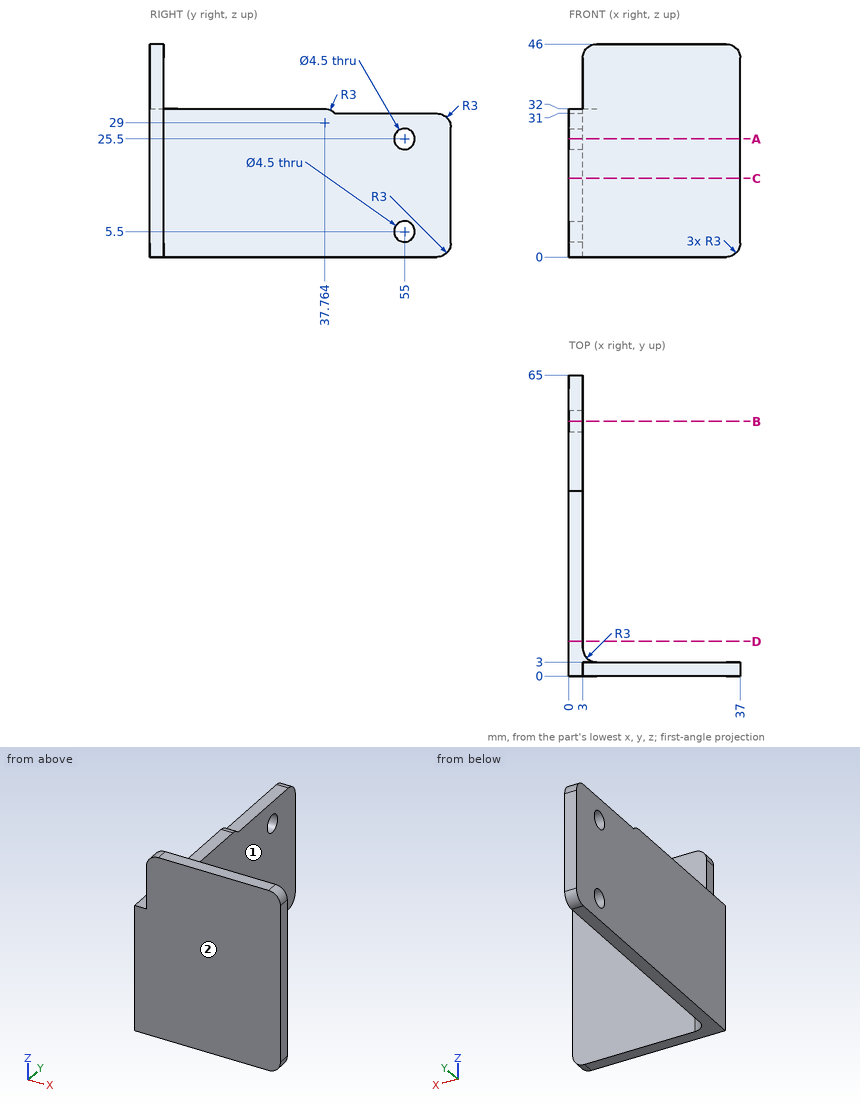
The drawing under review shows one solid part. Ordinate dimensions are in mm from its lowest x, y, z. A direction names the side the tool comes from. Coordinates: 2 decimals unless noted, no trailing zeros. Order: outer loops, then holes, each group sorted by start corner. A loop starts at its lowest first (then second) coordinate and runs counter-clockwise, first axis right, second up. Notation, with made-up numbers: (32.25, -22.75) -> (69.25, -22.75) arc R28 ccw to (69.25, 3.25) -> close; hole circle Ø8 at (-39.75, 23.25). An arc over 180 degrees is marked (long way). Answer as CSV lines item,"result".
Q1. We need section B-B (y = 55). State the section outline as (x, z) points.
Model answer:
outline,"(0, 0) -> (3, 0) -> (3, 3.25) -> (0, 3.25) -> close; (0, 7.75) -> (3, 7.75) -> (3, 23.25) -> (0, 23.25) -> close; (0, 27.75) -> (3, 27.75) -> (3, 31) -> (0, 31) -> close"
Q2. We need section D-D (y = 7.5). State the section outline as (x, z) points, plus the area to 3 significant figures.
Model answer:
outline,"(0, 0) -> (3, 0) -> (3, 32) -> (0, 32) -> close"
area,"96.0 mm2"
Q3. We need section C-C (z = 17). State the section outline as (x, y) points, plus the area to 3 significant figures.
Model answer:
outline,"(0, 0) -> (37, 0) -> (37, 3) -> (6, 3) arc R3 cw to (3, 6) -> (3, 65) -> (0, 65) -> close"
area,"299 mm2"
Q4. For the marked faces 1 and 2, list the 3-axis set-ups (+Z, -Z, +X, -X, +Y, -Y) from which the entire face can be reached by the end or side of a thin tool; tool diameter is ignored.
Model answer:
face 1,"+Z, -Z, +X, +Y"
face 2,"+Z, -Z, +X, -X, -Y"
Q5. We need section A-A (z = 25.5). State the section outline as (x, y) points, plus the area to 3 significant figures.
Model answer:
outline,"(0, 0) -> (37, 0) -> (37, 3) -> (6, 3) arc R3 cw to (3, 6) -> (3, 52.75) -> (0, 52.75) -> close; (0, 57.25) -> (3, 57.25) -> (3, 65) -> (0, 65) -> close"
area,"285 mm2"
Q6. Clearance check with flat-ended pins moving along their axes: pin 1 Ø10 at (x, z) = (27.5, 20) entering from -Y; pin 2 Ø4 at (y, z) = (55, 25.5) entering from +X; pin 3 Ø0.9 at (x, y) = (1, 46.5) entering from +Z; pin 4 Ø1.5 at (y, z) = (1, 40) entering from -X. State where each tip first meets the part, or that it passes through.
Model answer:
pin 1,"stops at y = 0"
pin 2,"passes through"
pin 3,"stops at z = 31"
pin 4,"stops at x = 3"
Q7. Wall thickness on line 1 along Z through (x, y) = (2.3, 55); line 2 along Y through (x, z) = (4.5, 37): over which ranges is each line inside the solid? List them lowest first. Write a range as [from, to].
Model answer:
line 1,"z = [0, 3.25], [7.75, 23.25], [27.75, 31]"
line 2,"y = [0, 3]"
